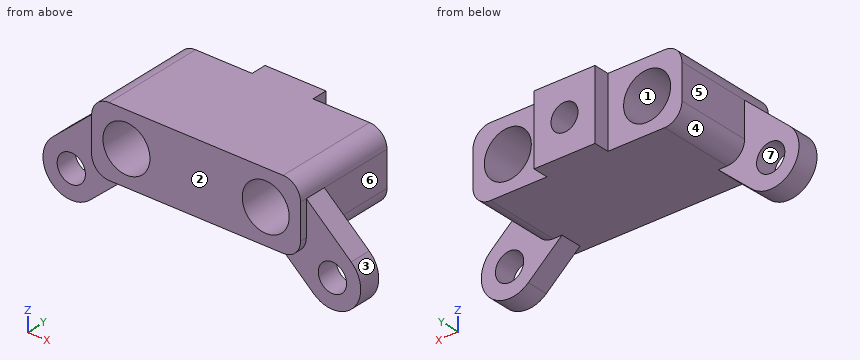
from build123d import *

# Parameters (mm, degrees)
SKETCH25_W          = 7
SKETCH25_H          = 8
BOSS_EXTRUDE5_DEPTH = 13.8
SKETCH26_W          = 24
SKETCH26_H          = 8
SKETCH26_R          = 2.7
BOSS_EXTRUDE6_DEPTH = 12
FILLET1_R           = 2
SKETCH27_R          = 1.55
CUT_EXTRUDE1_DEPTH  = 6.5
SKETCH29_R          = 1.625
BOSS_EXTRUDE8_DEPTH = 2.5


with BuildPart() as part:
    # Sketch25 → Boss-Extrude5 (new body)
    with BuildSketch(Plane(origin=(0, 0, 0), x_dir=(-1, 0, 0), z_dir=(0, 1, 0))):
        Rectangle(SKETCH25_W, SKETCH25_H)
    extrude(amount=BOSS_EXTRUDE5_DEPTH)

    # Sketch26 → Boss-Extrude6 (add)
    with BuildSketch(Plane(origin=(0, 0, 0), x_dir=(-1, 0, 0), z_dir=(0, 1, 0))):
        Rectangle(SKETCH26_W, SKETCH26_H)
        with Locations(Location((-8, 0, 0), (0, 0, 90))):
            Circle(SKETCH26_R, mode=Mode.SUBTRACT)
        with Locations(Location((8, 0, 0), (0, 0, 90))):
            Circle(SKETCH26_R, mode=Mode.SUBTRACT)
    extrude(amount=BOSS_EXTRUDE6_DEPTH)

    # Fillet1
    fillet1_edges = [part.edges().sort_by_distance(p)[0] for p in [
        (12, 6, -4),
        (-12, 6, 4),
        (12, 6, 4),
        (-12, 6, -4),
    ]]
    fillet(fillet1_edges, radius=FILLET1_R)

    # Sketch27 → Cut-Extrude1 (cut)
    with BuildSketch(Plane(origin=(0, 13.8, 0), x_dir=(1, 0, 0), z_dir=(0, 1, 0))):
        with Locations(Location((0, 0, 0), (0, 0, 270))):
            Circle(SKETCH27_R)
    extrude(amount=-CUT_EXTRUDE1_DEPTH, mode=Mode.SUBTRACT)

    # Sketch29 → Boss-Extrude8 (add)
    # profile 1 of 2: a face of its own
    with BuildSketch(Plane.XZ.offset(-0.8)):
        with BuildLine():
            Line((-17.155221844, -2.567404924), (-12, 2))
            Line((-12, 2), (-11, -3))
            Line((-11, -3), (-8.970414177, -4))
            Line((-8.970414177, -4), (-12.844778156, -7.432595076))
            ThreePointArc((-12.844778156, -7.432595076), (-17.432595076, -7.155221844), (-17.155221844, -2.567404924))
        make_face()
        with Locations(Location((-15, -5, 0), (0, 0, 270))):
            Circle(SKETCH29_R, mode=Mode.SUBTRACT)
    # profile 2 of 2: a face of its own
    with BuildSketch(Plane.XZ.offset(-0.8)):
        with BuildLine():
            Line((17.155221844, -2.567404924), (12, 2))
            Line((12, 2), (11, -3))
            Line((11, -3), (8.970414177, -4))
            Line((8.970414177, -4), (12.844778156, -7.432595076))
            ThreePointArc((12.844778156, -7.432595076), (17.432595076, -7.155221844), (17.155221844, -2.567404924))
        make_face()
        with Locations(Location((15, -5, 0), (0, 0, 90))):
            Circle(SKETCH29_R, mode=Mode.SUBTRACT)
    extrude(amount=-BOSS_EXTRUDE8_DEPTH)


solid = part.part
Geometry check sheet. Reference: the model listing, model coordinates, mm. Face numbers are marked on the shaded views. A direction names the side the tool comes from. Round coordinates to 2 decimals unless told otherwise and drop trailing zeros. Loops run counter-clockwise (first coordinate to the right, second up) from the corner with the lowest first, then second, coordinate; pieces in that order, holes last.
Item 1: Cross-section at B-B on x = -8. Record the boundary of the cut face in (y, z), then the cut area to 3 significant figures.
Item 2: Cross-section at A-A on y = 1.75. Record the boundary of the cut face in (x, z) (3 decimals), then the cut area to 3 significant figures.
Item 3: Mould release check, pull along Z, two halves, no side actions. Record for the marked faces 1, 2, 3 and 4: pulls with the +Z half, pulls with the -Z half, needs draft (parallel to the pull), parting line crosses it, or undercut.
Item 4: Cross-section at D-D on z = 1. Record the boundary of the cut face in (x, y), then the cut area to 3 significant figures.
Item 5: Cross-section at C-C on y = 4.75. Record the boundary of the cut face in (x, z).
Item 6: Access from +Z, -Z, +X, -X, +Y, -Y to the whole of each face (thin tool, end or side, straight path). Record for the marked faces 5, 6 and 7.
Item 7: Thickness scan on line 1 (X direction, y = 4.25, z = 0); line 2 (X direction, y = 2.5, z = 0); line 3 (X direction, y = 10.25, z = -0.75). Record the ranges inside material, lowest first.
Item 8: Gauge pin test, flat ends, axial feed: pin 1 (0.9 mm diameter, centred on x = 0.5, z = -0.5, fed in from +Y); pin 2 (1.2 mm diameter, centred on y = 6.5, z = 0, fed in from -X); pin 3 (5 mm diameter, centred on y = 11.5, z = -5.5, fed in from -X); pin 4 (6 mm diameter, centred on x = -13, z = -2.5, fed in from -Y). Record the tip position at first contact, or that the pin passes through.
Answer sheet:
1. outline: (0, -4) - (12, -4) - (12, -2.7) - (0, -2.7) - close; (0, 2.7) - (12, 2.7) - (12, 4) - (0, 4) - close
1. area: 31.2 mm2
2. outline: (-17.155, -2.567) arc R3.25 ccw to (-12.845, -7.433) - (-8.97, -4) - (8.97, -4) - (12.845, -7.433) arc R3.25 ccw to (17.155, -2.567) - (12, 2) arc R2 ccw to (10, 4) - (-10, 4) arc R2 ccw to (-12, 2) - close; hole circle Ø3.25 at (-15, -5); hole circle Ø5.4 at (-8, 0); hole circle Ø5.4 at (8, 0); hole circle Ø3.25 at (15, -5)
2. area: 221 mm2
3. face 1: undercut
3. face 2: needs draft
3. face 3: parting line crosses it
3. face 4: pulls with the -Z half
4. outline: (-13.13, 0.8) - (-12, 0.8) - (-12, 0) - (-10.51, 0) - (-10.51, 12) - (-12, 12) - (-12, 3.3) - (-13.13, 3.3) - close; (-5.49, 0) - (5.49, 0) - (5.49, 12) - (3.5, 12) - (3.5, 13.8) - (1.18, 13.8) - (1.18, 7.3) - (-1.18, 7.3) - (-1.18, 13.8) - (-3.5, 13.8) - (-3.5, 12) - (-5.49, 12) - close; (10.51, 0) - (12, 0) - (12, 0.8) - (13.13, 0.8) - (13.13, 3.3) - (12, 3.3) - (12, 12) - (10.51, 12) - close
4. area: 170 mm2
5. outline: (-12, -2) arc R2 ccw to (-10, -4) - (10, -4) arc R2 ccw to (12, -2) - (12, 2) arc R2 ccw to (10, 4) - (-10, 4) arc R2 ccw to (-12, 2) - close; hole circle Ø5.4 at (-8, 0); hole circle Ø5.4 at (8, 0)
6. face 5: +Z, -Z, -X, +Y
6. face 6: +Z, -Z, +X, +Y
6. face 7: +Y, -Y
7. line 1: x = -12 to -10.7, -5.3 to 5.3, 10.7 to 12
7. line 2: x = -14.26 to -10.7, -5.3 to 5.3, 10.7 to 14.26
7. line 3: x = -12 to -10.59, -5.41 to -1.36, 1.36 to 5.41, 10.59 to 12
8. pin 1: stops at y = 7.3
8. pin 2: stops at x = -12
8. pin 3: stops at x = -11.73
8. pin 4: stops at y = 0
